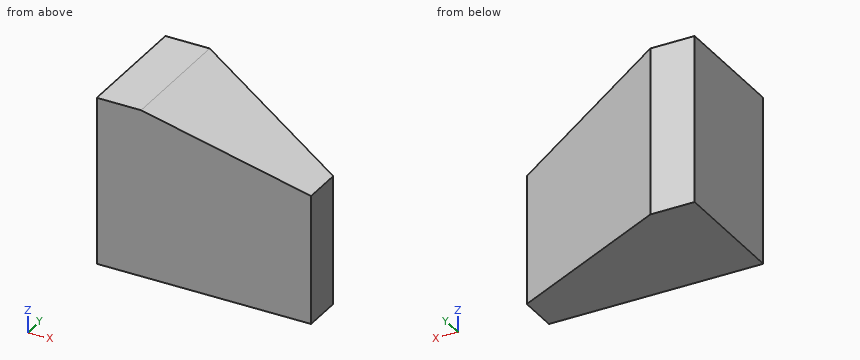
Autodesk Inventor part; units mm, degrees
ref_plane "YZ Plane" through (0, 0, 0) normal (1, 0, 0) x (0, 1, 0)
ref_plane "XZ Plane" through (0, 0, 0) normal (0, 1, 0) x (-1, 0, 0)
ref_plane "XY Plane" through (0, 0, 0) normal (0, 0, 1) x (1, 0, 0)
sketch "Sketch1" plane through (0, 0, 0) normal (0, 0, 1) x (1, 0, 0)
  line L0 (0, 0) -> (32.4623, 0)
  line L1 (32.4623, 0) -> (32.4623, 18.6079)
  line L2 (32.4623, 18.6079) -> (0, 18.6079)
  line L3 (0, 18.6079) -> (0, 0)
extrude "Extrusion1" add sketch "Sketch1" along normal blind 25.4
sketch "Sketch2" plane through (0, 0, 25.4) normal (0, 0, 1) x (1, 0, 0)
  line L0 (32.4623, 0) -> (32.4623, 18.6079)
  line L1 (32.4623, 18.6079) -> (0, 18.6079)
  line L2 (6.7125, 18.6079) -> (32.4623, 6.0135)
extrude "Extrusion2" cut sketch "Sketch2" against normal through all
sketch "Sketch3" plane through (0, 0, 0) normal (0, -1, 0) x (1, 0, 0)
  line L0 (32.4623, 0) -> (32.4623, 25.4)
  line L1 (0, 25.4) -> (32.4623, 25.4)
  line L2 (6.7125, 25.4) -> (6.7125, 0)
  line L3 (6.7125, 25.4) -> (32.4623, 19.5746)
extrude "Extrusion3" cut sketch "Sketch3" against normal through all
properties part number "Work Planes"
Part model, mm, in its own coordinate system. Coordinates: 2 decimals unless noted, no trailing zeros. Write each loop counter-clockwise with the first axis right and the second up, starting at its lowest first coordinate (ties: lowest second). Pieces come first, ordered by that corner, then holes. Notation, with made-up numbers: M 89,-3.75 L 106,-3.75 A13 cw 106,3.25 Z; hole C 4,-6 d4. An arc over 180 degrees is marked long. Return JSON: item names as keys, results as strings.
1. Saw through at D-D, the plane x = 7.5. Write the cut outline in (y, z).
Determined:
{"outline": "M 0,0 L 18.22,0 L 18.22,25.22 L 0,25.22 Z"}
2. Probe L1, parallel to Y at x = 10.5, z = 22.5; L2, parallel to X at y = 10.75, z = 6; L3, parallel to Y at x = 24, z = 1.5. List the from-to ranges inside material, lowest first.
Determined:
{"L1": "0 to 16.76", "L2": "0 to 22.78", "L3": "0 to 10.15"}
3. Saw through at C-C, the plane x = 29. Write the cut outline in (y, z), then the cut area to 3 significant figures.
Determined:
{"outline": "M 0,0 L 7.71,0 L 7.71,20.36 L 0,20.36 Z", "area": "157 mm²"}
4. Flat gauge pins, fed straight in: pin 1 Ø5 at (x, y) = (15, 12) entering from +Z; pin 2 Ø6 at (x, y) = (23.5, 5) entering from +Z; pin 3 Ø12 at (x, z) = (25.5, 16.5) entering from +Y. Where does each tip first touch, or does it go through?
Determined:
{"pin 1": "z = 24.09", "pin 2": "z = 22.28", "pin 3": "y = 12.35"}
5. Saw through at A-A, the plane y = 1.25. Write the cut outline in (x, z), then the cut area to 3 significant figures.
Determined:
{"outline": "M 0,0 L 32.46,0 L 32.46,19.57 L 6.71,25.4 L 0,25.4 Z", "area": "750 mm²"}
6. Saw through at B-B, the plane z = 4.25. Write the cut outline in (x, y), then the cut area to 3 significant figures.
Determined:
{"outline": "M 0,0 L 32.46,0 L 32.46,6.01 L 6.71,18.61 L 0,18.61 Z", "area": "442 mm²"}
